Design review of the part built by this model. Coordinates are the model's own, in mm. Face numbers are marked on the shaded views. A direction names the side the tool comes from. Give positions to 0.01 mm unless a question says otherwise; leave off trailing zeros. Loops run counter-clockwise (first coordinate to the right, second up) from the corner with the lowest first, then second, coordinate; pieces in that order, holes last. Notation, with made-up numbers: (27.25, 67.25) -> (74.25, 67.25) arc R17 ccw to (74.25, 98.25) -> close; hole circle Ø8 at (82, 74.25). An arc over 180 degrees is marked (long way). Use a Markdown table: item, result. Add a question column.
1. For the marked faces 1 and 2, list the 3-axis set-ups (+Z, -Z, +X, -X, +Y, -Y) from which the entire face can be reached by the end or side of a thin tool; tool diameter is ignored.
2. Add section B-B (y = 0.95). Count the separate pieces of the cut face and the enclosed holes in it, and give its area (3 significant figures).
3. For pin 1 Ø1.7 at (x, z) = (12, -1.5) entering from +Y; pin 2 Ø1.5 at (y, z) = (1.5, -2.5) entering from +X; pin 3 Ø4 at (x, z) = (0, 0) entering from +Y, all flat-tipped, find the tip position at first contact; note any pin that passes through.
4. Add section C-C (x = 12.5). State the section outline as (y, z) points.
5. To check wall thickness, follow line 1 (X direction, y = 2.3, z = 0); line 2 (Y direction, x = -7, z = 2); line 3 (X direction, y = 4.3, z = -1.5). State the ranges of each line that lie inside material, in increasing order.
6. Add section D-D (x = -8.5). State the section outline as (y, z) points, and give its area (3 significant figures).
7. Draft analysis for pull direction Z (two halves, no side actions). For the marked faces 3, 4 and 5, state which applies: pulls with the +Z half, pulls with the -Z half, needs draft (parallel to the pull), parting line crosses it, or undercut.
8. Add section A-A (x = 0). State the section outline as (y, z) points.
```python
from build123d import *

# Parameters (mm, degrees)
BOSS_EXTRUDE1_DEPTH = 2
SKETCH5_R           = 0.5
CUT_EXTRUDE5_DEPTH  = 3
LPATTERN1_COUNT     = 6
LPATTERN1_PITCH     = 2
MIRROR2_OUTLINE_R   = 0.5
MIRROR2_DEPTH       = 2
SKETCH2_R           = 3.75
BOSS_EXTRUDE2_DEPTH = 4.5
SKETCH3_R           = 2.25
CUT_EXTRUDE1_DEPTH  = 3
SKETCH4_R           = 1.4
CUT_EXTRUDE2_DEPTH  = 3


# Read off the part's stored shape, not the designer's step: Mirror2
with BuildPart() as part:
    # Sketch1 → Boss-Extrude1 (new body)
    with BuildSketch(Plane(origin=(0, 0, 0), x_dir=(1, 0, 0), z_dir=(0, 1, 0))):
        with BuildLine():
            Line((0, 3), (14.136480176, 2))
            ThreePointArc((14.136480176, 2), (15.461917194, 1.366812545), (16, 0))
            Line((16, 0), (0, 0))
            Line((0, 0), (0, 3))
        make_face()
    boss_extrude1 = extrude(amount=BOSS_EXTRUDE1_DEPTH)

    # Mirror1: Boss-Extrude1 across plane
    add(boss_extrude1.mirror(Plane.XY))

    # Sketch5 → Cut-Extrude5 (cut)
    with BuildSketch(Plane(origin=(0, 0, 0), x_dir=(1, 0, 0), z_dir=(0, 1, 0))):
        with Locations(Location((4.5, 0, 0), (0, 0, 90))):
            Circle(SKETCH5_R)
    cut_extrude5 = extrude(amount=CUT_EXTRUDE5_DEPTH, mode=Mode.SUBTRACT)

    # LPattern1: Cut-Extrude5 ×6
    with Locations(*[(i * LPATTERN1_PITCH, 0, 0) for i in range(1, LPATTERN1_COUNT)]):
        add(cut_extrude5, mode=Mode.SUBTRACT)

    # Mirror2 outline → Mirror2 (add)
    with BuildSketch(Plane(origin=(0, 0, 0), x_dir=(1, 0, 0), z_dir=(0, 1, 0))):
        with BuildLine():
            Line((0, -3), (0, 3))
            Line((0, 3), (-14.136480176, 2))
            ThreePointArc((-14.136480176, 2), (-16, 0), (-14.136480176, -2))
            Line((-14.136480176, -2), (0, -3))
        make_face()
        with Locations((-14.5, 0)):
            Circle(MIRROR2_OUTLINE_R, mode=Mode.SUBTRACT)
        with Locations((-12.5, 0)):
            Circle(MIRROR2_OUTLINE_R, mode=Mode.SUBTRACT)
        with Locations((-10.5, 0)):
            Circle(MIRROR2_OUTLINE_R, mode=Mode.SUBTRACT)
        with Locations((-8.5, 0)):
            Circle(MIRROR2_OUTLINE_R, mode=Mode.SUBTRACT)
        with Locations((-6.5, 0)):
            Circle(MIRROR2_OUTLINE_R, mode=Mode.SUBTRACT)
        with Locations((-4.5, 0)):
            Circle(MIRROR2_OUTLINE_R, mode=Mode.SUBTRACT)
    extrude(amount=MIRROR2_DEPTH)

    # Sketch2 → Boss-Extrude2 (add)
    with BuildSketch(Plane(origin=(0, 0, 0), x_dir=(1, 0, 0), z_dir=(0, 1, 0))):
        with Locations(Location((0, 0, 0), (0, 0, 48.893793678))):
            Circle(SKETCH2_R)
    extrude(amount=BOSS_EXTRUDE2_DEPTH)

    # Sketch3 → Cut-Extrude1 (cut)
    with BuildSketch(Plane(origin=(0, 4.5, 0), x_dir=(1, 0, 0), z_dir=(0, 1, 0))):
        with Locations(Location((0, 0, 0), (0, 0, 270))):
            Circle(SKETCH3_R)
    extrude(amount=-CUT_EXTRUDE1_DEPTH, mode=Mode.SUBTRACT)

    # Sketch4 → Cut-Extrude2 (cut)
    with BuildSketch(Plane(origin=(0, 1.5, 0), x_dir=(1, 0, 0), z_dir=(0, 1, 0))):
        with Locations(Location((0, 0, 0), (0, 0, 270))):
            Circle(SKETCH4_R)
    extrude(amount=-CUT_EXTRUDE2_DEPTH, mode=Mode.SUBTRACT)


solid = part.part
```
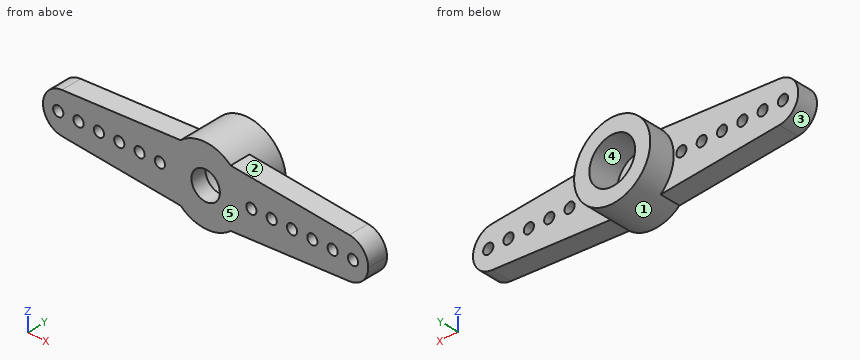
Taken from the geometry:
| question | item | result |
|---|---|---|
| 1 | face 1 | +Y |
| 1 | face 2 | +Z, +X, +Y, -Y |
| 2 | separate pieces | 1 |
| 2 | enclosed holes | 13 |
| 2 | area | 143 mm^2 |
| 3 | pin 1 | stops at y = 2 |
| 3 | pin 2 | stops at x = 14.97 |
| 3 | pin 3 | stops at y = 1.5 |
| 4 | outline | (0, -2.12) -> (2, -2.12) -> (2, -0.5) -> (0, -0.5) -> close; (0, 0.5) -> (2, 0.5) -> (2, 2.12) -> (0, 2.12) -> close |
| 5 | line 1 | x = -3.75 to -2.25, 2.25 to 3.75 |
| 5 | line 2 | y = 0 to 2 |
| 5 | line 3 | x = -3.44 to -1.68, 1.68 to 3.44 |
| 6 | outline | (0, -2.4) -> (2, -2.4) -> (2, -0.5) -> (0, -0.5) -> close; (0, 0.5) -> (2, 0.5) -> (2, 2.4) -> (0, 2.4) -> close |
| 6 | area | 7.59 mm^2 |
| 7 | face 3 | parting line crosses it |
| 7 | face 4 | undercut |
| 7 | face 5 | needs draft |
| 8 | outline | (0, -3.75) -> (4.5, -3.75) -> (4.5, -2.25) -> (1.5, -2.25) -> (1.5, -1.4) -> (0, -1.4) -> close; (0, 1.4) -> (1.5, 1.4) -> (1.5, 2.25) -> (4.5, 2.25) -> (4.5, 3.75) -> (0, 3.75) -> close |
